The model under review builds one solid part; all positions refer to its coordinate system, in mm. A direction names the side the tool comes from. Give positions to 0.01 mm unless a question says otherwise; leave off trailing zeros.
```python
from build123d import *

# Parameters (mm, degrees)
EXTRUDE_2_DEPTH     = 100
SKETCH_1_R          = 2
CUT_EXTRUDE_1_DEPTH = 143.439460825
SKETCH_2_R          = 2
CUT_EXTRUDE_2_DEPTH = 143.439460825


with BuildPart() as part:
    # 17F200L100 → ﾎﾞｽ - 押し出し2 (new body)
    with BuildSketch(Plane.XY):
        with BuildLine():
            Line((-98, 4), (-94, 4))
            Line((-94, 4), (-93.749844059, 16.265293393))
            ThreePointArc((-93.749844059, 16.265293393), (-93, 17), (-92.250155941, 16.265293393))
            Line((-92.250155941, 16.265293393), (-92, 4))
            Line((-92, 4), (-88, 4))
            Line((-88, 4), (-87.749844059, 16.265293393))
            ThreePointArc((-87.749844059, 16.265293393), (-87, 17), (-86.250155941, 16.265293393))
            Line((-86.250155941, 16.265293393), (-86, 4))
            Line((-86, 4), (-82, 4))
            Line((-82, 4), (-81.749844059, 16.265293393))
            ThreePointArc((-81.749844059, 16.265293393), (-81, 17), (-80.250155941, 16.265293393))
            Line((-80.250155941, 16.265293393), (-80, 4))
            Line((-80, 4), (-76, 4))
            Line((-76, 4), (-75.749844059, 16.265293393))
            ThreePointArc((-75.749844059, 16.265293393), (-75, 17), (-74.250155941, 16.265293393))
            Line((-74.250155941, 16.265293393), (-74, 4))
            Line((-74, 4), (-70, 4))
            Line((-70, 4), (-69.749844059, 16.265293393))
            ThreePointArc((-69.749844059, 16.265293393), (-69, 17), (-68.250155941, 16.265293393))
            Line((-68.250155941, 16.265293393), (-68, 4))
            Line((-68, 4), (-64, 4))
            Line((-64, 4), (-63.749844059, 16.265293393))
            ThreePointArc((-63.749844059, 16.265293393), (-63, 17), (-62.250155941, 16.265293393))
            Line((-62.250155941, 16.265293393), (-62, 4))
            Line((-62, 4), (-58, 4))
            Line((-58, 4), (-57.749844059, 16.265293393))
            ThreePointArc((-57.749844059, 16.265293393), (-57, 17), (-56.250155941, 16.265293393))
            Line((-56.250155941, 16.265293393), (-56, 4))
            Line((-56, 4), (-52, 4))
            Line((-52, 4), (-51.749844059, 16.265293393))
            ThreePointArc((-51.749844059, 16.265293393), (-51, 17), (-50.250155941, 16.265293393))
            Line((-50.250155941, 16.265293393), (-50, 4))
            Line((-50, 4), (-46, 4))
            Line((-46, 4), (-45.749844059, 16.265293393))
            ThreePointArc((-45.749844059, 16.265293393), (-45, 17), (-44.250155941, 16.265293393))
            Line((-44.250155941, 16.265293393), (-44, 4))
            Line((-44, 4), (-40, 4))
            Line((-40, 4), (-39.749844059, 16.265293393))
            ThreePointArc((-39.749844059, 16.265293393), (-39, 17), (-38.250155941, 16.265293393))
            Line((-38.250155941, 16.265293393), (-38, 4))
            Line((-38, 4), (-34, 4))
            Line((-34, 4), (-33.749844059, 16.265293393))
            ThreePointArc((-33.749844059, 16.265293393), (-33, 17), (-32.250155941, 16.265293393))
            Line((-32.250155941, 16.265293393), (-32, 4))
            Line((-32, 4), (-28, 4))
            Line((-28, 4), (-27.749844059, 16.265293393))
            ThreePointArc((-27.749844059, 16.265293393), (-27, 17), (-26.250155941, 16.265293393))
            Line((-26.250155941, 16.265293393), (-26, 4))
            Line((-26, 4), (-22, 4))
            Line((-22, 4), (-21.749844059, 16.265293393))
            ThreePointArc((-21.749844059, 16.265293393), (-21, 17), (-20.250155941, 16.265293393))
            Line((-20.250155941, 16.265293393), (-20, 4))
            Line((-20, 4), (-16, 4))
            Line((-16, 4), (-15.749844059, 16.265293393))
            ThreePointArc((-15.749844059, 16.265293393), (-15, 17), (-14.250155941, 16.265293393))
            Line((-14.250155941, 16.265293393), (-14, 4))
            Line((-14, 4), (-10, 4))
            Line((-10, 4), (-9.749844059, 16.265293393))
            ThreePointArc((-9.749844059, 16.265293393), (-9, 17), (-8.250155941, 16.265293393))
            Line((-8.250155941, 16.265293393), (-8, 4))
            Line((-8, 4), (-4, 4))
            Line((-4, 4), (-3.749844059, 16.265293393))
            ThreePointArc((-3.749844059, 16.265293393), (-3, 17), (-2.250155941, 16.265293393))
            Line((-2.250155941, 16.265293393), (-2, 4))
            Line((-2, 4), (2, 4))
            Line((2, 4), (2.250155941, 16.265293393))
            ThreePointArc((2.250155941, 16.265293393), (3, 17), (3.749844059, 16.265293393))
            Line((3.749844059, 16.265293393), (4, 4))
            Line((4, 4), (8, 4))
            Line((8, 4), (8.250155941, 16.265293393))
            ThreePointArc((8.250155941, 16.265293393), (9, 17), (9.749844059, 16.265293393))
            Line((9.749844059, 16.265293393), (10, 4))
            Line((10, 4), (14, 4))
            Line((14, 4), (14.250155941, 16.265293393))
            ThreePointArc((14.250155941, 16.265293393), (15, 17), (15.749844059, 16.265293393))
            Line((15.749844059, 16.265293393), (16, 4))
            Line((16, 4), (20, 4))
            Line((20, 4), (20.250155941, 16.265293393))
            ThreePointArc((20.250155941, 16.265293393), (21, 17), (21.749844059, 16.265293393))
            Line((21.749844059, 16.265293393), (22, 4))
            Line((22, 4), (26, 4))
            Line((26, 4), (26.250155941, 16.265293393))
            ThreePointArc((26.250155941, 16.265293393), (27, 17), (27.749844059, 16.265293393))
            Line((27.749844059, 16.265293393), (28, 4))
            Line((28, 4), (32, 4))
            Line((32, 4), (32.250155941, 16.265293393))
            ThreePointArc((32.250155941, 16.265293393), (33, 17), (33.749844059, 16.265293393))
            Line((33.749844059, 16.265293393), (34, 4))
            Line((34, 4), (38, 4))
            Line((38, 4), (38.250155941, 16.265293393))
            ThreePointArc((38.250155941, 16.265293393), (39, 17), (39.749844059, 16.265293393))
            Line((39.749844059, 16.265293393), (40, 4))
            Line((40, 4), (44, 4))
            Line((44, 4), (44.250155941, 16.265293393))
            ThreePointArc((44.250155941, 16.265293393), (45, 17), (45.749844059, 16.265293393))
            Line((45.749844059, 16.265293393), (46, 4))
            Line((46, 4), (50, 4))
            Line((50, 4), (50.250155941, 16.265293393))
            ThreePointArc((50.250155941, 16.265293393), (51, 17), (51.749844059, 16.265293393))
            Line((51.749844059, 16.265293393), (52, 4))
            Line((52, 4), (56, 4))
            Line((56, 4), (56.250155941, 16.265293393))
            ThreePointArc((56.250155941, 16.265293393), (57, 17), (57.749844059, 16.265293393))
            Line((57.749844059, 16.265293393), (58, 4))
            Line((58, 4), (62, 4))
            Line((62, 4), (62.250155941, 16.265293393))
            ThreePointArc((62.250155941, 16.265293393), (63, 17), (63.749844059, 16.265293393))
            Line((63.749844059, 16.265293393), (64, 4))
            Line((64, 4), (68, 4))
            Line((68, 4), (68.250155941, 16.265293393))
            ThreePointArc((68.250155941, 16.265293393), (69, 17), (69.749844059, 16.265293393))
            Line((69.749844059, 16.265293393), (70, 4))
            Line((70, 4), (74, 4))
            Line((74, 4), (74.250155941, 16.265293393))
            ThreePointArc((74.250155941, 16.265293393), (75, 17), (75.749844059, 16.265293393))
            Line((75.749844059, 16.265293393), (76, 4))
            Line((76, 4), (80, 4))
            Line((80, 4), (80.250155941, 16.265293393))
            ThreePointArc((80.250155941, 16.265293393), (81, 17), (81.749844059, 16.265293393))
            Line((81.749844059, 16.265293393), (82, 4))
            Line((82, 4), (86, 4))
            Line((86, 4), (86.250155941, 16.265293393))
            ThreePointArc((86.250155941, 16.265293393), (87, 17), (87.749844059, 16.265293393))
            Line((87.749844059, 16.265293393), (88, 4))
            Line((88, 4), (92, 4))
            Line((92, 4), (92.250155941, 16.265293393))
            ThreePointArc((92.250155941, 16.265293393), (93, 17), (93.749844059, 16.265293393))
            Line((93.749844059, 16.265293393), (94, 4))
            Line((94, 4), (98, 4))
            Line((98, 4), (98.250155941, 16.265293393))
            ThreePointArc((98.250155941, 16.265293393), (99, 17), (99.749844059, 16.265293393))
            Line((99.749844059, 16.265293393), (100, 4))
            Line((100, 4), (100, 0))
            Line((100, 0), (-100, 0))
            Line((-100, 0), (-100, 4))
            Line((-100, 4), (-99.749844059, 16.265293393))
            ThreePointArc((-99.749844059, 16.265293393), (-99, 17), (-98.250155941, 16.265293393))
            Line((-98.250155941, 16.265293393), (-98, 4))
        make_face()
    extrude(amount=EXTRUDE_2_DEPTH)

    # ｽｹｯﾁ1 → ｶｯﾄ - 押し出し1 (cut, through all)
    with BuildSketch(Plane.XZ):
        with Locations(Location((-78, 50, 0), (0, 0, 270))):
            Circle(SKETCH_1_R)
        with Locations(Location((90, 50, 0), (0, 0, 270))):
            Circle(SKETCH_1_R)
    extrude(amount=-CUT_EXTRUDE_1_DEPTH, mode=Mode.SUBTRACT)

    # ｽｹｯﾁ2 → ｶｯﾄ - 押し出し2 (cut, through all)
    with BuildSketch(Plane(origin=(0, 0, 0), x_dir=(-1, 0, 0), z_dir=(0, -1, 0))):
        with Locations(Location((48, -85, 0), (0, 0, 90))):
            Circle(SKETCH_2_R)
        with Locations(Location((48, -15, 0), (0, 0, 90))):
            Circle(SKETCH_2_R)
        with Locations(Location((90, -85, 0), (0, 0, 90))):
            Circle(SKETCH_2_R)
        with Locations(Location((90, -15, 0), (0, 0, 90))):
            Circle(SKETCH_2_R)
    extrude(amount=-CUT_EXTRUDE_2_DEPTH, mode=Mode.SUBTRACT)


solid = part.part
```
Item 1: Take a section at A-A (y = 9). Give the number of separate pieces and of enclosed holes in the cut face, and give its area (3 significant figures).
Values found:
separate pieces: 34
enclosed holes: 0
area: 6,110 mm2
Item 2: Clearance check with flat-ended pins moving along their axes: pin 1 Ø1.2 at (x, z) = (-54.5, 36) entering from +Y; pin 2 Ø1 at (x, z) = (14.5, 66.5) entering from +Y. State where each tip first meets the part, or that it passes through.
Values found:
pin 1: stops at y = 4
pin 2: stops at y = 17
Item 3: For faces 1 (the cylindrical face through (-88.314, 1.972, 83.925)), 2 (the flat face through (6, 4, 49)), list the 3-axis set-ups (+Z, -Z, +X, -X, +Y, -Y) from which the entire face can be reached by the end or side of a thin tool; tool diameter is ignored.
Values found:
face 1: +Y, -Y
face 2: +Z, -Z, +Y
Item 4: For line 1 (X direction, y = 2.25, z = 85); line 2 (X direction, y = 1.95, z = 50); line 3 (Z direction, x = -48, y = 2.75), list the stretches that pass through material, from the lowest coordinate up.
Values found:
line 1: x = -100 to -92, -88 to -50, -46 to 100
line 2: x = -100 to -80, -76 to 88, 92 to 100
line 3: z = 0 to 13, 17 to 83, 87 to 100
